Input: part model. Units: mm. Frame: model coordinates. Face numbers are marked on the shaded views. A direction names the side the tool comes from. Coordinates: 2 decimals unless noted, no trailing zeros. Loops run counter-clockwise (first coordinate to the right, second up) from the corner with the lowest first, then second, coordinate; pieces in that order, holes last. Notation, with made-up numbers: (53.5, 89) - (94.5, 89) arc R9 cw to (94.5, 104) - close; hole circle Ø7 at (60, 70.25). An arc over 180 degrees is marked (long way). Answer as CSV lines item,"result". Start each with the question number.
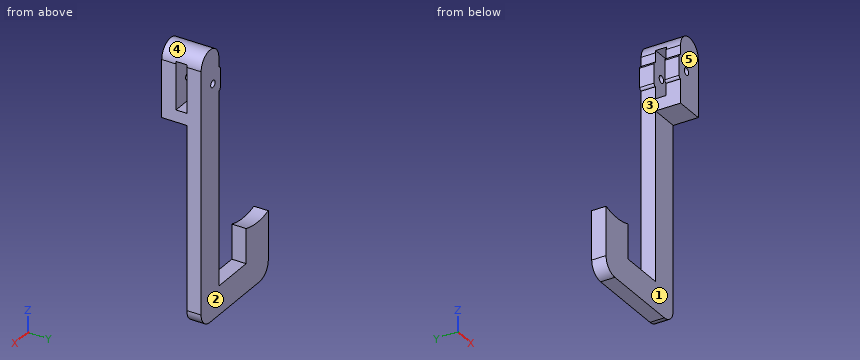
```python
from build123d import *

# Parameters (mm, degrees)
BOSS_EXTRUDE1_DEPTH = 3
SKETCH2_R           = 12
CUT_EXTRUDE1_DEPTH  = 3
SKETCH5_W           = 6
SKETCH5_H           = 2.5
BOSS_EXTRUDE2_DEPTH = 5.25
SKETCH6_W           = 6
SKETCH6_H           = 3
BOSS_EXTRUDE3_DEPTH = 10
CUT_EXTRUDE2_REACH  = 54.879
SKETCH4_R           = 0.75
FILLET1_R           = 3
SKETCH8_W           = 0.5
SKETCH8_H           = 5
BOSS_EXTRUDE4_DEPTH = 3
FILLET2_R           = 0.5


# Some blends are built 0.0001 mm under size
with BuildPart() as part:
    # Sketch1 → Boss-Extrude1 (new body)
    with BuildSketch(Plane(origin=(0, 0, 0), x_dir=(1, 0, 0), z_dir=(0, 1, 0))):
        Polygon((-2, -7.5), (4, -7.5), (4, 48.75), (-18.75, 48.75), (-18.75, 28.369317262), (-11.25, 28.369317262), (-11.25, 42.75), (-2, 42.75), (-2, 2.5), (-2.5, 2.5), (-2.5, -2.5), (-2, -2.5), align=None)
    extrude(amount=BOSS_EXTRUDE1_DEPTH)

    # Sketch2 → Cut-Extrude1 (cut)
    with BuildSketch(Plane(origin=(0, 3, 0), x_dir=(1, 0, 0), z_dir=(0, 1, 0))):
        with Locations((-15.091915752, 24.129582051)):
            Circle(SKETCH2_R)
    extrude(amount=-CUT_EXTRUDE1_DEPTH, mode=Mode.SUBTRACT)

    # Sketch5 → Boss-Extrude2 (add)
    with BuildSketch(Plane.XZ):
        with Locations((1, -6.25)):
            Rectangle(SKETCH5_W, SKETCH5_H)
        with Locations((1, 6.25)):
            Rectangle(SKETCH5_W, SKETCH5_H)
    extrude(amount=BOSS_EXTRUDE2_DEPTH)

    # Sketch6 → Boss-Extrude3 (add)
    with BuildSketch(Plane(origin=(0, 0, 5), x_dir=(-1, 0, 0), z_dir=(0, 0, -1))):
        with Locations((-1, -3.75)):
            Rectangle(SKETCH6_W, SKETCH6_H)
    extrude(amount=BOSS_EXTRUDE3_DEPTH)

    # Cut-Extrude2: up to this face of the body (flat: up to its plane)
    cut_extrude2_end = Plane(part.part.faces().sort_by_distance((1, -5.25, 0))[0])
    # Sketch4 → Cut-Extrude2 (cut, up to the picked face)
    with BuildSketch(Plane(origin=(0, 3, 0), x_dir=(1, 0, 0), z_dir=(0, 1, 0)), mode=Mode.PRIVATE) as cut_extrude2_sk1:
        with Locations(Location((0, 0, 0), (0, 0, 90))):
            Circle(SKETCH4_R)
    cut_extrude2_tool1 = split(extrude(cut_extrude2_sk1.sketch, amount=-CUT_EXTRUDE2_REACH, mode=Mode.PRIVATE), bisect_by=cut_extrude2_end, keep=Keep.BOTH, mode=Mode.PRIVATE)
    add(cut_extrude2_tool1.solids().sort_by(Axis((0, 3, 0), (0, -1, 0)))[0], mode=Mode.SUBTRACT)

    # Fillet1
    # the kernel refuses this fillet: 3 mm, written as the material it takes off along each edge
    with BuildSketch(Plane(origin=(-18.75, -7.5, -48.75), x_dir=(1, 0, 0), z_dir=(0, 1, 0)), Plane(origin=(4, -7.5, -48.75), x_dir=(0, 0, 1), z_dir=(0, 1, 0))) as fillet1_piece_1:
        with BuildLine():
            CenterArc((FILLET1_R, -FILLET1_R), FILLET1_R, 90, 90)
            Line((0, -FILLET1_R), (0, 0))
            Line((0, 0), (FILLET1_R, 0))
        make_face()
    extrude(amount=18, mode=Mode.SUBTRACT)
    with BuildSketch(Plane(origin=(4, -12.75, 7.5), x_dir=(-1, 0, 0), z_dir=(0, 1, 0)), Plane(origin=(-2, -12.75, 7.5), x_dir=(0, 0, -1), z_dir=(0, 1, 0))) as fillet1_piece_2:
        with BuildLine():
            CenterArc((FILLET1_R, -FILLET1_R), FILLET1_R, 90, 90)
            Line((0, -FILLET1_R), (0, 0))
            Line((0, 0), (FILLET1_R, 0))
        make_face()
    extrude(amount=23.25, mode=Mode.SUBTRACT)

    # Sketch8 → Boss-Extrude4 (add)
    with BuildSketch(Plane(origin=(0, -2.25, 0), x_dir=(1, 0, 0), z_dir=(0, 1, 0))):
        with Locations((-2.25, 0)):
            Rectangle(SKETCH8_W, SKETCH8_H)
    extrude(amount=-BOSS_EXTRUDE4_DEPTH)

    # Fillet2
    fillet2_edges = [part.edges().sort_by_distance(p)[0] for p in [
        (-2.5, 1.5, 2.5),
        (-2.5, 1.5, -2.5),
        (-2.5, -3.75, 2.5),
        (-2.5, -3.75, -2.5),
    ]]
    fillet(fillet2_edges, radius=FILLET2_R - 0.0001)  # a hair under: the kernel refuses the full size


solid = part.part
```
Item 1: Set-up query: the marked faces 1 and 2. Return all of +Z, -Z, +X, -X, +Y, -Y with unobstructed straight access to the full face (end or side cutting, diameter ignored); none if empty.
Item 2: Section query A-A, the plane z = -38.5. Output: boundary loops of the cut face in (x, y), and give its area (3 significant figures).
Item 3: Section query D-D, the plane z = 0. Output: boundary loops of the cut face in (x, y), and give its area (3 significant figures).
Item 4: Material intervals for probe 1 along X at (y, z) = (0.9, 0); probe 2 along Y at (x, z) = (2.5, -10.5); probe 3 along Z at (x, y) = (-2.25, 0.5), sorted ascending.
Item 5: Contact query for flat-ended pins moving along their axis: P1, Ø0.9, axis at x = -5.5, y = 2, coming from the +Z side; P2, Ø0.9, axis at x = 0, z = 0, coming from the -Y side; P3, Ø2.5, axis at y = -3.5, z = -0.5, coming from the -X side; P4, Ø3, axis at y = 2, z = -16, coming from the -X side. Output: stop coordinate, or through.
Item 6: Section query B-B, the plane y = -1.75. Output: boundary loops of the cut face in (x, z).
Item 7: Draft query along X for the marked faces 3, 4 and 5. Return one class per face: pulls with the +X half, pulls with the -X half, needs draft (parallel to the pull), parting line crosses it, or undercut.
Response values:
1,face 1,"-Z, +X, -X, -Y"
1,face 2,"+Z, -Z, +X, -X, +Y"
2,outline,"(-18.75, 0) - (-11.25, 0) - (-11.25, 3) - (-18.75, 3) - close; (-2, 0) - (4, 0) - (4, 3) - (-2, 3) - close"
2,area,"40.5 mm²"
3,outline,"(-2.5, -5.25) - (-0.75, -5.25) - (-0.75, -2.25) - (-2.5, -2.25) - close; (-2.5, 0) - (-0.75, 0) - (-0.75, 3) - (-2.5, 3) - close; (0.75, -5.25) - (4, -5.25) - (4, -2.25) - (0.75, -2.25) - close; (0.75, 0) - (4, 0) - (4, 3) - (0.75, 3) - close"
3,area,"30.0 mm²"
4,probe 1,"x = -2.5 to -0.75, 0.75 to 4"
4,probe 2,"y = 0 to 3"
4,probe 3,"z = -48.75 to -42.75, -2.43 to 2.43"
5,P1,"stops at z = -42.75"
5,P2,"passes through"
5,P3,"stops at x = -2.5"
5,P4,"stops at x = -2"
6,outline,"(-2, -7.5) - (4, -7.5) - (4, -5) - (-2, -5) - close; (-1.96, 5) - (3.96, 5) arc R3 ccw to start"
7,face 3,"undercut"
7,face 4,"parting line crosses it"
7,face 5,"needs draft"
